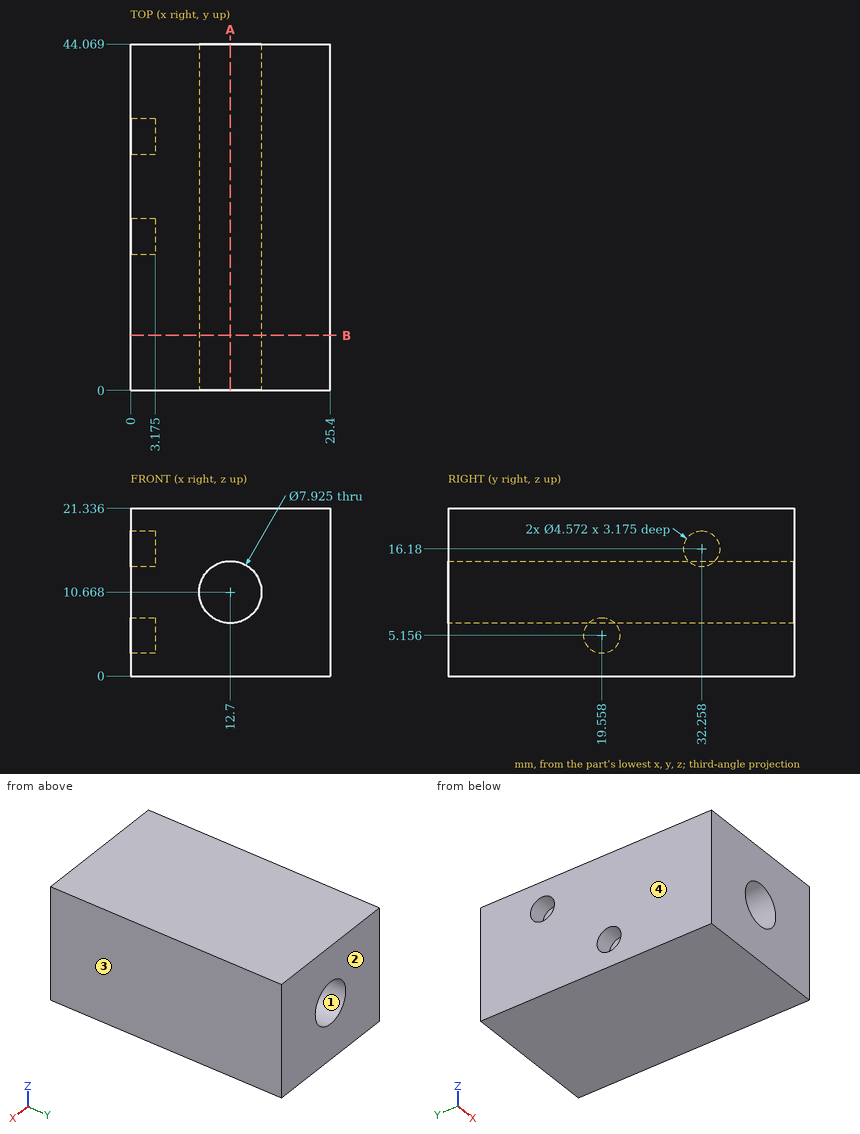
Check sheet for the drawn part. Datum: minimum x, y, z corner. Units: mm. Give positions to 0.01 mm unless a question says otherwise; leave off trailing zeros. Order: outer loops, then holes, each group sorted by start corner. A loop starts at its lowest first (then second) coordinate and runs counter-clockwise, first axis right, second up. Notation, with made-up numbers: (31.25, 18.5) -> (83.25, 18.5) arc R20 cw to (83.25, 27.5) -> close; hole circle Ø9 at (-11.75, -15.75). An arc over 180 degrees is marked (long way). Answer as CSV lines item,"result".
Q1. Sectioned sample at B-B on y = 7. Record the cut outline in (x, z) (1 decimal).
Solutions:
outline,"(0, 0) -> (25.4, 0) -> (25.4, 21.3) -> (0, 21.3) -> close; hole circle Ø7.9 at (12.7, 10.7)"
Q2. Depth check by flat-ended pin: pin 1 (3.5 mm diameter, centred on y = 19.56, z = 5.16, fed in from -X) (3 decimals); pin 2 (7 mm diameter, centred on x = 12.7, z = 10.668, fed in from -Y). Enter the tip coordinate at first touch or a pass-through.
Solutions:
pin 1,"stops at x = 3.175"
pin 2,"passes through"
Q3. Scan lines: probe 1 along Z at (x, y) = (13, 8.5); probe 2 along X at (y, z) = (12, 10.5); probe 3 along X at (y, z) = (27.5, 8). Record each from-to range of solid material in increasing order.
Solutions:
probe 1,"z = 0 to 6.72, 14.62 to 21.34"
probe 2,"x = 0 to 8.74, 16.66 to 25.4"
probe 3,"x = 0 to 9.77, 15.63 to 25.4"
Q4. Sectioned sample at A-A on x = 12.7. Record the cut outline in (y, z).
Solutions:
outline,"(0, 0) -> (44.07, 0) -> (44.07, 6.71) -> (0, 6.71) -> close; (0, 14.63) -> (44.07, 14.63) -> (44.07, 21.34) -> (0, 21.34) -> close"
Q5. Release check for a two-part mould opening along X. For the marked faces 1, 2, 3 and 4 record: +X half, -X half, draft (parallel to the pull), parting line (faces both ways), or undercut.
Solutions:
face 1,"undercut"
face 2,"draft"
face 3,"+X half"
face 4,"-X half"
